```python
from build123d import *

# Parameters (mm, degrees)
BOSS_EXTRUDE1_DEPTH         = 25.4
F_1_4_0_25_DIAMETER_HOLE1_D = 6.35
CHAMFER1_SIZE               = 7.9375
SKETCH6_R                   = 7.9375
CUT_EXTRUDE1_DEPTH          = 10.525


with BuildPart() as part:
    # Sketch1 → Boss-Extrude1 (new body)
    with BuildSketch(Plane.XY):
        with BuildLine():
            Line((6.35, 12.7), (31.75, 12.7))
            Line((31.75, 12.7), (31.75, 7.9375))
            Line((31.75, 7.9375), (15.875, 7.9375))
            Line((15.875, 7.9375), (15.875, -7.9375))
            Line((15.875, -7.9375), (31.75, -7.9375))
            Line((31.75, -7.9375), (31.75, -12.7))
            Line((31.75, -12.7), (6.35, -12.7))
            Line((6.35, -12.7), (6.35, -10.998522628))
            ThreePointArc((6.35, -10.998522628), (12.7, 0), (6.35, 10.998522628))
            Line((6.35, 10.998522628), (6.35, 12.7))
        make_face()
    extrude(amount=BOSS_EXTRUDE1_DEPTH)

    # 1/4 (0.25) Diameter Hole1 (through all)
    with Locations(Plane(origin=(0, 12.7, 0), x_dir=(1, 0, 0), z_dir=(0, 1, 0))):
        with Locations((25.4, -12.821774192)):
            Hole(F_1_4_0_25_DIAMETER_HOLE1_D / 2)

    # Chamfer1
    chamfer1_edges = [part.edges().sort_by_distance(p)[0] for p in [
        (31.75, 10.31875, 0),
        (31.75, 10.31875, 25.4),
        (31.75, -10.31875, 25.4),
        (31.75, -10.31875, 0),
    ]]
    chamfer(chamfer1_edges, length=CHAMFER1_SIZE)

    # Sketch6 → Cut-Extrude1 (cut, through all)
    with BuildSketch(Plane(origin=(15.875, 0, 0), x_dir=(0, 0, -1), z_dir=(1, 0, 0))):
        with Locations((-12.7, 0)):
            Circle(SKETCH6_R)
    extrude(amount=-CUT_EXTRUDE1_DEPTH, mode=Mode.SUBTRACT)


solid = part.part
```
Can you work these out from the model? Positions are in its coordinate system, mm. A direction names the side the tool comes from. Round coordinates to 2 decimals unless told otherwise and drop trailing zeros. Loops run counter-clockwise (first coordinate to the right, second up) from the corner with the lowest first, then second, coordinate; pieces in that order, holes last.
Item 1: Please list where these lines run through material, in increasing order: L1, parallel to Y at x = 21.5, z = 18.5; L2, parallel to Z at x = 13.25, y = 0; L3, parallel to Z at x = 13.25, y = 5.25.
Item 2: Will these pins go through, and if not, where does the flat tip stop? pin 1 Ø6.5 at (y, z) = (3.5, 5.5) entering from +X (3 decimals); pin 2 Ø4 at (x, z) = (23.5, 14) entering from +Y; pin 3 Ø4 at (x, z) = (25.4, 12.82) entering from +Y; pin 4 Ø2 at (y, z) = (9, 19.5) entering from -X.
Item 3: If we mould it in two halves opening along X, with no side actions, what happens to faces 3 (the flat face through (19, 12.7, 13)), 4 (the cylindrical face through (22.37, -10.35, 11.87)), 5 (the flat face through (6.35, -12, 13))? For each: +X half, -X half, draft (parallel to the pull), parting line (faces both ways), or undercut.
Item 4: Suppose I cut it at C-C, the plane x = 14.25. Write out the boundary of the cut face in (y, z) (1 decimal), then the cut area to 3 significant figures.
Item 5: Which directions (+Z, -Z, +X, -X, +Y, -Y) give clear straight access to the entire face, cutting with the end or side of a thin tool? Please do faces 1 (the flat face through (22, -7.938, 13)), 2 (the flat face through (15, 0, 25.4)).
Item 6: Suppose I cut it at B-B, the plane x = 8.5. Write out the boundary of the cut face in (y, z).
Item 7: Suppose I cut it at A-A, the plane y = 0. Write out the boundary of the cut face in (x, z) (1 decimal), then the cut area to 3 significant figures.
Reported:
1. L1: y = -12.7 to -7.94, 7.94 to 12.7
1. L2: z = 0 to 4.76, 20.64 to 25.4
1. L3: z = 0 to 6.75, 18.65 to 25.4
2. pin 1: stops at x = 15.875
2. pin 2: stops at y = 12.7
2. pin 3: passes through
2. pin 4: stops at x = 7.83
3. face 3: draft
3. face 4: undercut
3. face 5: -X half
4. outline: (-12.7, 0) - (12.7, 0) - (12.7, 25.4) - (-12.7, 25.4) - close; hole circle Ø15.9 at (0, 12.7)
4. area: 447 mm2
5. face 1: +Z, -Z, +X
5. face 2: +Z, +X, -X, +Y, -Y
6. outline: (-12.7, 0) - (-9.44, 0) - (-9.44, 25.4) - (-12.7, 25.4) - close; (9.44, 0) - (12.7, 0) - (12.7, 25.4) - (9.44, 25.4) - close
7. outline: (12.7, 0) - (15.9, 0) - (15.9, 4.8) - (12.7, 4.8) - close; (12.7, 20.6) - (15.9, 20.6) - (15.9, 25.4) - (12.7, 25.4) - close
7. area: 30.2 mm2
